Read the model definition and answer for the solid it produces. Units are mm, in the model's axes. Coordinates: 2 decimals unless noted, no trailing zeros. Order: outer loops, then holes, each group sorted by start corner. A loop starts at its lowest first (then second) coordinate and runs counter-clockwise, first axis right, second up. Notation, with made-up numbers: (80.5, 38) - (108.5, 38) arc R31 cw to (108.5, 77) - close; hole circle Ø7 at (-11, 77.25). An arc over 180 degrees is marked (long way). Use one line per item in the form item = value.
```python
from build123d import *

# Parameters (mm, degrees)
F1_DEPTH = 3.048


with BuildPart() as f1:
    # F0 (on Front) → F1 (new body)
    with BuildSketch(Plane.XZ):
        with BuildLine():
            Line((0, 79.375), (0, 104.775))
            ThreePointArc((0, 104.775), (-7.14375, 107.9998046905), (-9.4502929642, 115.490625))
            Line((-9.4502929642, 115.490625), (-15.7504882737, 65.484375))
            ThreePointArc((-15.7504882737, 65.484375), (-10.5003255158, 75.40625), (0, 79.375))
        make_face()
        with BuildLine():
            ThreePointArc((9.525, 114.3), (6.7351920908, 107.5648079092), (0, 104.775))
            Line((0, 104.775), (0, 79.375))
            ThreePointArc((0, 79.375), (10.5003255158, 75.40625), (15.7504882737, 65.484375))
            Line((15.7504882737, 65.484375), (9.4502929642, 115.490625))
            ThreePointArc((9.4502929642, 115.490625), (9.5063048942, 114.896483242), (9.525, 114.3))
        make_face()
        with BuildLine():
            ThreePointArc((15.7504882737, 65.484375), (10.5003255158, 75.40625), (0, 79.375))
            Line((0, 79.375), (0, 47.625))
            ThreePointArc((0, 47.625), (10.6492737428, 51.7267849017), (15.7954255641, 61.9125))
            ThreePointArc((15.7954255641, 61.9125), (15.8550939106, 62.7052534459), (15.875, 63.5))
            ThreePointArc((15.875, 63.5), (15.8438414904, 64.4941387366), (15.7504882737, 65.484375))
        make_face()
        with BuildLine():
            Line((0, 47.625), (0, 79.375))
            ThreePointArc((0, 79.375), (-10.5003255158, 75.40625), (-15.7504882737, 65.484375))
            ThreePointArc((-15.7504882737, 65.484375), (-15.8737438155, 63.6997054867), (-15.7954255641, 61.9125))
            ThreePointArc((-15.7954255641, 61.9125), (-10.6492737428, 51.7267849017), (0, 47.625))
        make_face()
        with BuildLine():
            Line((0, 9.525), (0, 47.625))
            ThreePointArc((0, 47.625), (-10.6492737428, 51.7267849017), (-15.7954255641, 61.9125))
            Line((-15.7954255641, 61.9125), (-9.4772553384, -0.9525))
            ThreePointArc((-9.4772553384, -0.9525), (-7.063929059, 6.3895642457), (0, 9.525))
        make_face()
        with BuildLine():
            ThreePointArc((-9.4502929642, 115.490625), (-7.14375, 107.9998046905), (0, 104.775))
            ThreePointArc((0, 104.775), (6.7351920908, 107.5648079092), (9.525, 114.3))
            ThreePointArc((9.525, 114.3), (9.5063048942, 114.896483242), (9.4502929642, 115.490625))
            ThreePointArc((9.4502929642, 115.490625), (0, 123.825), (-9.4502929642, 115.490625))
        make_face()
        with BuildLine():
            ThreePointArc((3.175, 114.3), (2.2450640303, 112.0549359697), (0, 111.125))
            ThreePointArc((0, 111.125), (-2.2450640303, 116.5450640303), (3.175, 114.3))
        make_face(mode=Mode.SUBTRACT)
        with BuildLine():
            ThreePointArc((71.9691688256, 0), (69.7134786398, 5.5426476963), (64.228458656, 7.935060177))
            ThreePointArc((64.228458656, 7.935060177), (58.4890211293, 5.6818098142), (56.0941688256, 0))
            ThreePointArc((56.0941688256, 0), (58.4890211293, -5.6818098142), (64.228458656, -7.935060177))
            ThreePointArc((64.228458656, -7.935060177), (69.7134786398, -5.5426476963), (71.9691688256, 0))
        make_face()
        with BuildLine():
            ThreePointArc((67.2066688256, 0), (64.0316688256, -3.175), (60.8566688256, 0))
            ThreePointArc((60.8566688256, 0), (64.0316688256, 3.175), (67.2066688256, 0))
        make_face(mode=Mode.SUBTRACT)
        with BuildLine():
            ThreePointArc((15.7954255641, 61.9125), (10.6492737428, 51.7267849017), (0, 47.625))
            Line((0, 47.625), (0, 9.525))
            ThreePointArc((0, 9.525), (0.1180829727, 9.524268025), (0.2361477965, 9.5220722124))
            Line((0.2361477965, 9.5220722124), (10.5043958672, 9.2674192228))
            Line((10.5043958672, 9.2674192228), (15.7954255641, 61.9125))
        make_face()
        with BuildLine():
            Line((10.5043958672, 9.2674192228), (0.2361477965, 9.5220722124))
            ThreePointArc((0.2361477965, 9.5220722124), (6.818171777, 6.6511772356), (9.525, 0))
            Line((9.525, 0), (9.5729851903, 0))
            Line((9.5729851903, 0), (10.5043958672, 9.2674192228))
        make_face()
        with BuildLine():
            ThreePointArc((9.4772553384, -0.9525), (6.4766458983, -6.9841737456), (0.2361477965, -9.5220722124))
            Line((0.2361477965, -9.5220722124), (64.228458656, -7.935060177))
            ThreePointArc((64.228458656, -7.935060177), (58.4890211293, -5.6818098142), (56.0941688256, 0))
            Line((56.0941688256, 0), (9.5729851903, 0))
            Line((9.5729851903, 0), (9.4772553384, -0.9525))
        make_face()
        with BuildLine():
            Line((0, 3.175), (0, 9.525))
            ThreePointArc((0, 9.525), (-7.063929059, 6.3895642457), (-9.4772553384, -0.9525))
            ThreePointArc((-9.4772553384, -0.9525), (-6.3015005456, -7.1425986779), (0.2361477965, -9.5220722124))
            ThreePointArc((0.2361477965, -9.5220722124), (6.4766458983, -6.9841737456), (9.4772553384, -0.9525))
            ThreePointArc((9.4772553384, -0.9525), (9.5130563464, -0.4768479324), (9.525, 0))
            Line((9.525, 0), (3.175, 0))
            ThreePointArc((3.175, 0), (-2.2450640303, -2.2450640303), (0, 3.175))
        make_face()
        with BuildLine():
            ThreePointArc((0.2361477965, 9.5220722124), (0.1180829727, 9.524268025), (0, 9.525))
            Line((0, 9.525), (0, 3.175))
            ThreePointArc((0, 3.175), (2.2450640303, 2.2450640303), (3.175, 0))
            Line((3.175, 0), (9.525, 0))
            ThreePointArc((9.525, 0), (6.818171777, 6.6511772356), (0.2361477965, 9.5220722124))
        make_face()
        with BuildLine():
            Line((64.228458656, 7.935060177), (10.5043958672, 9.2674192228))
            Line((10.5043958672, 9.2674192228), (9.5729851903, 0))
            Line((9.5729851903, 0), (56.0941688256, 0))
            ThreePointArc((56.0941688256, 0), (58.4890211293, 5.6818098142), (64.228458656, 7.935060177))
        make_face()
    extrude(amount=F1_DEPTH)


solid = f1.part
```
(1) Section A-A, the plane y = -2.4 is taken. State how many separate pieces and enclosed holes the cut face has, then the cut area to 3 significant figures.
Answer list:
separate_pieces = 1
enclosed_holes = 4
area = 4,160 mm2
(2) Section B-B, the plane x = 39 is taken. Write down the section's boundary in (y, z), then the cut area to 3 significant figures.
Answer list:
outline = (-3.05, -8.56) - (0, -8.56) - (0, 8.56) - (-3.05, 8.56) - close
area = 52.2 mm2
(3) Straight lines are drawn through the part: L1, parallel to Z at x = 0, y = -0.8 (3 decimals); L2, parallel to X at y = -1.75, z = 114.3 (3 decimals); L3, parallel to Z at x = 24.5, y = -0.8. For each, find the intervals that lie inside material, in ascending order.
Answer list:
L1 = -9.525 to -3.175, 3.175 to 111.125, 117.475 to 123.825
L2 = -9.6 to -3.175, 3.175 to 9.6
L3 = -8.92 to 8.92
(4) Section C-C, the plane z = 72 is taken. Write down the section's boundary in (x, y).
Answer list:
outline = (-14.93, -3.05) - (14.93, -3.05) - (14.93, 0) - (-14.93, 0) - close
(5) The mould has two halves that part along Z. Classify faces 1 (the flat face through (-12.68, -1.5, 30.92)), 2 (the flat face through (12, -3.048, 43)), 3 (the flat face through (-12.556, -1.503, 90.838)), 4 (the flat face through (13.113, -1.503, 35.221)): +Z half, -Z half, draft (parallel to the pull), parting line (faces both ways), or undercut.
Answer list:
face_1 = -Z half
face_2 = draft
face_3 = +Z half
face_4 = undercut
(6) Given pin 1 Ø1.5 at (y, z) = (-2, 106.5) entering from +X, flat-ended and moving along its own axis, determine where the tip first touches the part or whether it passes through.
Answer list:
pin_1 = 10.68
